Here's how the part is built. I have some questions about the finished solid (model axes, mm). Face numbers are marked on the shaded views. Round coordinates to 2 decimals unless told otherwise and drop trailing zeros. Write each loop counter-clockwise with the first axis right and the second up, starting at its lowest first coordinate (ties: lowest second). Pieces come first, ordered by that corner, then holes. Notation, with made-up numbers: (4.5, 63) - (39.5, 63) arc R20 cw to (39.5, 100) - close; hole circle Ø8 at (-2.75, 18.25). An arc over 180 degrees is marked (long way). One line per item, written item: value. Start each with the question number.
Item 1: Imagine slicing it at B-B, the plane z = 4. Count the separate pieces of the cut face and the enclosed holes in it, then the cut area to 3 significant figures.
Item 2: If I drill on line 1 (Y direction, x = -0.5, z = 4.5); line 2 (X direction, y = 2, z = 2.5); line 3 (X direction, y = 2.5, z = 1.75), over which ranges is the centre line in solid material (lowest first)?
Item 3: Imagine slicing it at A-A, the plane y = 0. Please give me the cut outline in (x, z), then the cut area to 3 significant figures.
Item 4: Imagine slicing it at C-C, the plane x = 6.75. Please give me the cut outline in (y, z).
Item 5: For P1, Ø2, axis at y = -21, z = 1, coming from the -X side; P2, Ø1.5, axis at y = -15.5, z = 1, coming from the +X side; P3, Ø6.5, axis at x = 0, y = 0, coming from the +Z side; P4, Ø1, axis at y = -19, z = 2, coming from the +X side (3 decimals), each with a flat end and sliding along its axis, tell me the tip position at first contact or that it passes through.
Item 6: Thinking about a two-plate mould opening in X: for the marked faces 1, 2 and 3, which applies, released by +X, released by -X, zero draft, split by the parting line, or undercut?
Item 7: Imagine slicing it at D-D, the plane y = 8. Please give me the cut outline in (x, z), then the cut area to 3 significant figures.
```python
from build123d import *

# Parameters (mm, degrees)
SKETCH1_R           = 4
SKETCH1_R_2         = 1.75
BOSS_EXTRUDE1_DEPTH = 6.35


with BuildPart() as part:
    # Sketch1 → Boss-Extrude1 (new body)
    with BuildSketch(Plane.XY):
        with BuildLine():
            ThreePointArc((-11.077287152, -0.883948864), (0, 11.1125), (11.077287152, -0.883948864))
            ThreePointArc((11.077287152, -0.883948864), (9.32030962, -11.480690637), (5.802388508, -21.6296875))
            ThreePointArc((5.802388508, -21.6296875), (3.459876036, -24.374636871), (0, -25.4))
            ThreePointArc((0, -25.4), (-3.459876036, -24.374636871), (-5.802388508, -21.6296875))
            ThreePointArc((-5.802388508, -21.6296875), (-9.32030962, -11.480690637), (-11.077287152, -0.883948864))
        make_face()
        Circle(SKETCH1_R, mode=Mode.SUBTRACT)
        with Locations((8, 0)):
            Circle(SKETCH1_R_2, mode=Mode.SUBTRACT)
        with Locations((0, -8)):
            Circle(SKETCH1_R_2, mode=Mode.SUBTRACT)
        with Locations((-8, 0)):
            Circle(SKETCH1_R_2, mode=Mode.SUBTRACT)
        with Locations((0, 8)):
            Circle(SKETCH1_R_2, mode=Mode.SUBTRACT)
    extrude(amount=BOSS_EXTRUDE1_DEPTH)


solid = part.part
```
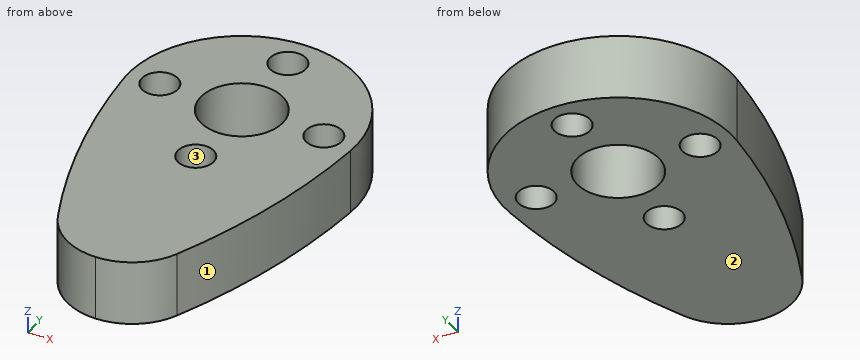
Values follow:
1. separate pieces: 1
1. enclosed holes: 5
1. area: 532 mm^2
2. line 1: y = -25.38 to -9.68, -6.32 to -3.97, 3.97 to 6.32, 9.68 to 11.1
2. line 2: x = -10.93 to -3.46, 3.46 to 10.93
2. line 3: x = -10.83 to -3.12, 3.12 to 10.83
3. outline: (-11.11, 0) - (-9.75, 0) - (-9.75, 6.35) - (-11.11, 6.35) - close; (-6.25, 0) - (-4, 0) - (-4, 6.35) - (-6.25, 6.35) - close; (4, 0) - (6.25, 0) - (6.25, 6.35) - (4, 6.35) - close; (9.75, 0) - (11.11, 0) - (11.11, 6.35) - (9.75, 6.35) - close
3. area: 45.9 mm^2
4. outline: (-19.38, 0) - (-1.22, 0) - (-1.22, 6.35) - (-19.38, 6.35) - close; (1.22, 0) - (8.83, 0) - (8.83, 6.35) - (1.22, 6.35) - close
5. P1: stops at x = -6.5
5. P2: stops at x = 8.4
5. P3: passes through
5. P4: stops at x = 7.095
6. face 1: released by +X
6. face 2: zero draft
6. face 3: undercut
7. outline: (-7.71, 0) - (-1.75, 0) - (-1.75, 6.35) - (-7.71, 6.35) - close; (1.75, 0) - (7.71, 0) - (7.71, 6.35) - (1.75, 6.35) - close
7. area: 75.7 mm^2
